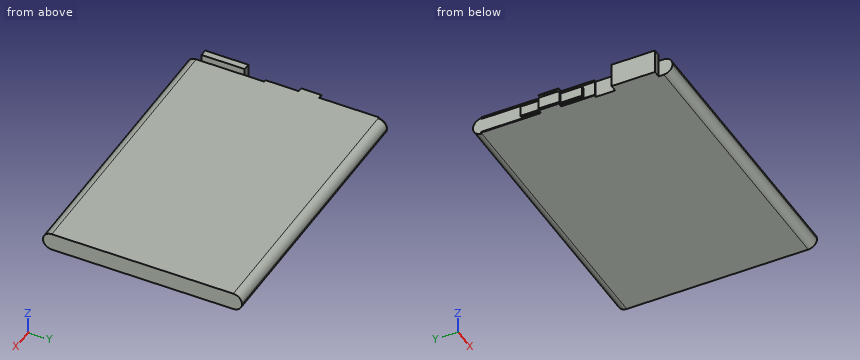
Autodesk Fusion 360 part; units mm, degrees
sketch "Sketch1" plane through (0, 0, 0) normal (0, 0, 1) x (1, 0, 0)
  line L0 (0, 0) -> (79.58, 0)
  line L1 (79.58, 0) -> (79.58, 57)
  line L2 (79.58, 57) -> (0, 57)
  line L3 (0, 57) -> (0, 0)
  dimension "d1" = 79.58
  dimension "d2" = 57
extrude "Extrude1" add sketch "Sketch1" along normal blind 5
fillet "Fillet1" radius 2.5 4 edges at (39.79, 0, 5) (39.79, 0, 0) (39.79, 57, 5) (39.79, 57, 0)
sketch "Sketch2" plane through (0, 0, 0) normal (-1, 0, 0) x (0, -1, 0)
  arc A0 (-54.5, 5) -> (-54.5, 0) centre (-54.5, 2.5) ccw
  line L0 (-54.5, 0) -> (-2.5, 0)
  arc A1 (-2.5, 0) -> (-2.5, 5) centre (-2.5, 2.5) ccw
  line L1 (-2.5, 5) -> (-54.5, 5)
  line L2 (-54.5, 5) -> (-22, 5)
  line L3 (-22, 5) -> (-22, 0)
  line L4 (-22, 0) -> (-54.5, 0)
  arc A2 (-54.5, 5) -> (-54.5, 0) centre (-54.5, 2.5) ccw
  dimension "d7" = 5
  dimension "d8" = 32.5
extrude "Extrude2" add sketch "Sketch2" along normal blind 0.3 contours A0 L0 L1 L2 L3 L4 A2
sketch "Sketch4" plane through (-0.3, 0, 0) normal (-1, 0, 0) x (0, -1, 0)
  line L0 (-22, 5) -> (-54.5, 5)
  arc A0 (-54.5, 5) -> (-54.5, 0) centre (-54.5, 2.5) ccw
  line L1 (-54.5, 0) -> (-22, 0)
  line L2 (-22, 0) -> (-22, 5)
  line L3 (-54.5, 0) -> (-22, 0)
  line L4 (-22, 0) -> (-22, 0.25)
  line L5 (-22, 0.25) -> (-54.5, 0.25)
  line L6 (-54.5, 0.25) -> (-54.5, 0)
  line L7 (-59.156, 2.5) -> (0.7958, 2.5) construction
  line L8 (-54.5, 5) -> (-22, 5)
  line L9 (-22, 5) -> (-22, 4.75)
  line L10 (-22, 4.75) -> (-54.5, 4.75)
  line L11 (-54.5, 4.75) -> (-54.5, 5)
  dimension "d11" = 0.25
extrude "Extrude3" add sketch "Sketch4" along normal blind 0.35 contours L0 L2 L8 L9 L10 L11 | L1 L2 L3 L4 L5 L6
sketch "Sketch5" plane through (-0.65, 0, 0) normal (-1, 0, 0) x (0, -1, 0)
  line L0 (-54.5, 0) -> (-22, 0)
  line L1 (-22, 0) -> (-22, 0.25)
  line L2 (-31.55, 0.25) -> (-37.35, 0.25)
  line L3 (-37.35, 0.25) -> (-37.35, 0)
  line L4 (-37.35, 0) -> (-31.55, 0)
  line L5 (-31.55, 0) -> (-31.55, 0.25)
  line L6 (-54.5, 0.25) -> (-54.5, 0)
  line L7 (-22, 0.25) -> (-54.5, 0.25)
  line L8 (-58.264, 2.5) -> (4.0505, 2.5) construction
  line L9 (-22, 5) -> (-54.5, 5) construction
  line L10 (-31.55, 4.75) -> (-37.35, 4.75)
  line L11 (-37.35, 4.75) -> (-37.35, 5)
  line L12 (-37.35, 5) -> (-31.55, 5)
  line L13 (-31.55, 5) -> (-31.55, 4.75)
  dimension "d18" = 5.8
  dimension "d19" = 2.5
  dimension "d20" = 2.5
extrude "Extrude4" add sketch "Sketch5" along normal blind 1.25 contours L0 L2 L3 L4 L5 L7 | L10 L11 L12 L13
sketch "Sketch6" plane through (0, 0, 0) normal (-1, 0, 0) x (0, -1, 0)
  line L0 (-22, 5) -> (-22, 0)
  line L1 (-22, 0) -> (-2.5, 0)
  arc A0 (-2.5, 0) -> (-2.5, 5) centre (-2.5, 2.5) ccw
  line L2 (-2.5, 5) -> (-22, 5)
  line L3 (-4, 7) -> (-16.4, 7)
  line L4 (-16.4, 7) -> (-16.4, 0)
  line L5 (-16.4, 0) -> (-4, 0)
  line L6 (-4, 0) -> (-4, 7)
  line L7 (0, 8.6382) -> (0, -2.5126) construction
  dimension "d21" = 4
  dimension "d22" = 12.4
  dimension "d23" = 2
extrude "Extrude5" add sketch "Sketch6" along normal blind 2 contours L2 L3 L4 L6 | L1 L2 L4 L5 L6
sketch "Sketch7" plane through (-0.3, 0, 0) normal (-1, 0, 0) x (0, -1, 0)
  line L0 (-22, 4.75) -> (-54.5, 4.75)
  line L1 (-54.5, 4.75) -> (-54.5, 5)
  arc A0 (-54.5, 5) -> (-54.5, 0) centre (-54.5, 2.5) ccw
  line L2 (-54.5, 0) -> (-54.5, 0.25)
  line L3 (-54.5, 0.25) -> (-22, 0.25)
  line L4 (-22, 0.25) -> (-22, 4.75)
  line L5 (-37.55, 4.25) -> (-31.55, 4.25)
  line L6 (-31.55, 4.25) -> (-31.55, 0.75)
  line L7 (-31.55, 0.75) -> (-37.55, 0.75)
  line L8 (-37.55, 0.75) -> (-37.55, 4.25)
  line L9 (-59.3246, 2.5) -> (-29.1063, 2.5) construction
  line L10 (-31.55, 7.2978) -> (-31.55, -1.062) construction
  point P0 (-31.55, 5)
  dimension "d26" = 6
  dimension "d27" = 3.5
  dimension "d28" = 1.75
extrude "Extrude7" add sketch "Sketch7" along normal blind 1.4 contours L5 L6 L7 L8
sketch "Sketch8" plane through (-0.3, 0, 0) normal (-1, 0, 0) x (0, -1, 0)
  line L0 (-22, 4.75) -> (-54.5, 4.75)
  line L1 (-54.5, 4.75) -> (-54.5, 5)
  arc A0 (-54.5, 5) -> (-54.5, 0) centre (-54.5, 2.5) ccw
  line L2 (-54.5, 0) -> (-54.5, 0.25)
  line L3 (-54.5, 0.25) -> (-22, 0.25)
  line L4 (-22, 0.25) -> (-22, 4.75)
  line L5 (-25.4, 4) -> (-43.1, 4)
  line L6 (-43.1, 4) -> (-43.1, 1)
  line L7 (-43.1, 1) -> (-25.4, 1)
  line L8 (-25.4, 1) -> (-25.4, 4)
  line L9 (-57, 2.5) -> (-22, 2.5) construction
  line L10 (-37.55, 0.75) -> (-37.55, 4.25)
  line L11 (-37.55, 4.25) -> (-31.55, 4.25)
  line L12 (-31.55, 4.25) -> (-31.55, 0.75)
  line L13 (-31.55, 0.75) -> (-37.55, 0.75)
  dimension "d29" = 1.5
  dimension "d30" = 3
  dimension "d31" = 17.7
  dimension "d32" = 3.4
extrude "Extrude6" add sketch "Sketch8" along normal blind 0.65 contours L5 L7 L8 L12 | L5 L7 L10 L12 | L5 L6 L7 L10
equation "d8 = 35 mm - ( d7 / 2 )"
equation "d28 = d27 / 2"
equation "d29 = d30 / 2"
The model under review builds one solid part; all positions refer to its coordinate system, in mm. Give positions to 0.01 mm unless a question says otherwise; leave off trailing zeros. Write each loop counter-clockwise with the first axis right and the second up, starting at its lowest first coordinate (ties: lowest second). Pieces come first, ordered by that corner, then holes. Notation, with made-up numbers: (31, 35) -> (83, 35) arc R24 cw to (83, 64) -> close; hole circle Ø8 at (8, -24.75). An arc over 180 degrees is marked (long way). Answer in a Markdown table with one row per item.
1) Add section C-C on y = 15.5. State the section outline as (x, z) points, plus the area to 3 significant figures.
Worked answers:
| item | result |
|---|---|
| outline | (-2, 0) -> (79.58, 0) -> (79.58, 5) -> (0, 5) -> (0, 7) -> (-2, 7) -> close |
| area | 412 mm² |
2) Add section A-A on y = 48.5. State the section outline as (x, z) points, plus the area to 3 significant figures.
Worked answers:
| item | result |
|---|---|
| outline | (-0.65, 0) -> (79.58, 0) -> (79.58, 5) -> (-0.65, 5) -> (-0.65, 4.75) -> (-0.3, 4.75) -> (-0.3, 0.25) -> (-0.65, 0.25) -> close |
| area | 400 mm² |
3) For L1, parallel to X at y = 12, z = 5.75; L2, parallel to X at y = 17.5, z = 3.5; L3, parallel to Z at x = 74, y = 53, list the stretches that pass through material, from the lowest coordinate up. Write a range as [from, to].
Worked answers:
| item | result |
|---|---|
| L1 | [-2, 0] |
| L2 | [0, 79.58] |
| L3 | [0, 5] |
4) Clearance check with flat-ended pins moving along their axes: P1, Ø0.7, axis at x = -0.5, y = 29, coming from the +Z side; P2, Ø3.5, axis at y = 28, z = 2, coming from the -X side; P3, Ø0.5, axis at x = -0.5, z = 2, coming from the -Y side. State where each tip first meets the part, or that it passes through.
Worked answers:
| item | result |
|---|---|
| P1 | z = 5 |
| P2 | x = -0.95 |
| P3 | y = 4 |
